Print and shaded views of the part. All mm, measured from the part's lowest x, y and z. A direction names the side the tool comes from. Round coordinates to 2 decimals unless told otherwise and drop trailing zeros. Loops run counter-clockwise (first coordinate to the right, second up) from the corner with the lowest first, then second, coordinate; pieces in that order, holes last. Notation, with made-up numbers: M 77.5,5.25 L 84.5,5.25 A22 ccw 84.5,27.25 Z; hole C 56.5,15.5 d8. An arc over 180 degrees is marked long. One line per item, written item: value. Start each with the question number.
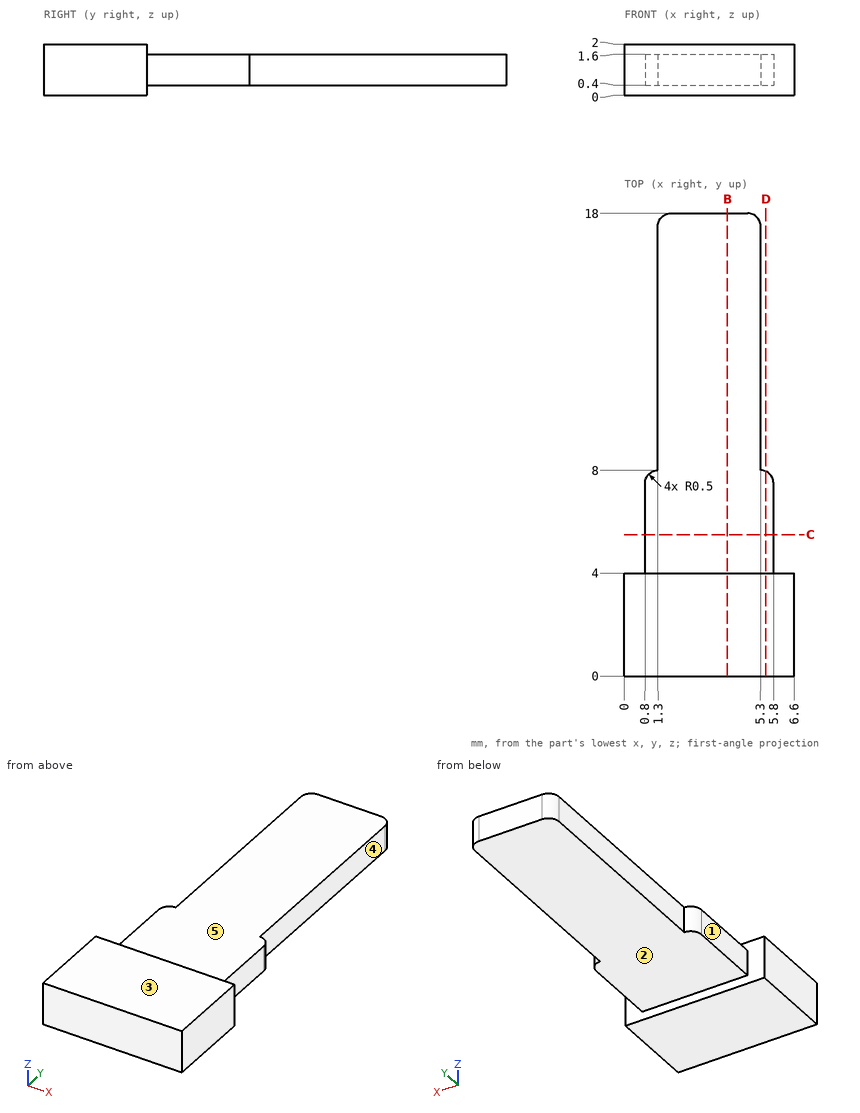
(1) Which spindle directions (+Z, -Z, +X, -X, +Y, -Y) get a long thin tool onto all of the face, cutting with end or side? Do the marked faces 1, 2, 3, 4 and 5. Say none if no direction does.
(2) Flat gauge pins, fed straight in: P1, Ø1, axis at y = 5, z = 1, coming from the +X side; P2, Ø3, axis at x = 2, y = 15.5, coming from the -Z side; P3, Ø1, axis at y = 15, z = 1, coming from the -X side. Where does each tip first touch, or does it go through?
(3) Slice it at B-B, the plane x = 4. List the corners of the cut face in (y, z), and give its area (3 significant figures).
(4) Slice it at C-C, the plane y = 5.5. List the corners of the cut face in (x, z).
(5) Probe L1, parallel to Y at x = 6.25, z = 0.15; L2, parallel to Z at x = 4.75, y = 4.75; L3, parallel to X at y = 6, z = 1.15. List the from-to ranges inside material, lowest first.
(6) Slice it at D-D, the plane x = 5.5. List the corners of the cut face in (y, z).
Check result:
1. face 1: +Z, -Z, -X, +Y
1. face 2: -Z, +X, -X, +Y
1. face 3: +Z, +X, -X, +Y, -Y
1. face 4: +Z, -Z, +X, +Y
1. face 5: +Z, +X, -X, +Y
2. P1: stops at x = 5.8
2. P2: stops at z = 0.4
2. P3: stops at x = 1.3
3. outline: M 0,0 L 4,0 L 4,0.4 L 18,0.4 L 18,1.6 L 4,1.6 L 4,2 L 0,2 Z
3. area: 24.8 mm^2
4. outline: M 0.8,0.4 L 5.8,0.4 L 5.8,1.6 L 0.8,1.6 Z
5. L1: y = 0 to 4
5. L2: z = 0.4 to 1.6
5. L3: x = 0.8 to 5.8
6. outline: M 0,0 L 4,0 L 4,0.4 L 7.96,0.4 L 7.96,1.6 L 4,1.6 L 4,2 L 0,2 Z
